Source: CAD feature listing. Evaluate the final solid. Frame: model axes, mm. A direction names the side the tool comes from. Give positions to 0.01 mm unless a question says otherwise; leave off trailing zeros. Loops run counter-clockwise (first coordinate to the right, second up) from the corner with the lowest first, then second, coordinate; pieces in that order, holes last. Notation, with made-up numbers: M -32,29.5 L -9,29.5 A20 ccw -9,40.5 Z; hole C 55.5,1.5 d5. An arc over 180 degrees is marked long. Put each result on its own line as item: value.
Autodesk Inventor part; units mm, degrees
ref_plane "YZ Plane" through (0, 0, 0) normal (1, 0, 0) x (0, 1, 0)
ref_plane "XZ Plane" through (0, 0, 0) normal (0, 1, 0) x (-1, 0, 0)
ref_plane "XY Plane" through (0, 0, 0) normal (0, 0, 1) x (1, 0, 0)
sketch "Sketch1" plane through (0, 0, 0) normal (1, 0, 0) x (0, 1, 0)
  arc A0 (43.0231, 66.0406) -> (13.0231, 66.0406) centre (28.0231, 66.0406) ccw
  arc A1 (13.0231, -33.9594) -> (43.0231, -33.9594) centre (28.0231, -33.9594) ccw
  line L0 (13.0231, 66.0406) -> (13.0231, -33.9594)
  line L1 (43.0231, 66.0406) -> (43.0231, -33.9594)
  circle A2 centre (28.0231, 66.0406) radius 5
  circle A3 centre (28.0231, -33.9594) radius 5
  circle A4 centre (28.0231, 36.0406) radius 2
  circle A5 centre (28.0231, -13.9594) radius 2
  point P0 (0, 0)
  dimension "d6" = 15
  dimension "d18" = 100
  dimension "d40" = 10
  dimension "d50" = 0
  dimension "d51" = 0
  dimension "d52" = 20
  dimension "d53" = 30
  dimension "d54" = 4
  dimension "d66" = 10
extrude "Extrusion6" add sketch "Sketch1" along normal blind 4
hole "Hole4" at (4, 28.0231, 66.0406) direction (-1, 0, 0) diameter 11.6 depth 0.8 tip angle 118
hole "Hole5" at (4, 28.0231, -33.9594) direction (-1, 0, 0) diameter 11.6 depth 0.8
properties part number "BaseJoint"
1. Section query A-A (x = 1.7). Output: boundary loops of the cut face in (y, z).
Found:
outline: M 13.02,-33.96 A15 ccw 43.02,-33.96 L 43.02,66.04 A15 ccw 13.02,66.04 Z; hole C 28.02,-33.96 d10; hole C 28.02,66.04 d10; hole C 28.02,-13.96 d4; hole C 28.02,36.04 d4
2. Contact query for flat-ended pins moving along their axis: P1, Ø2.5, axis at y = 28.02, z = 36.04, coming from the +X side; P2, Ø1.5, axis at x = 1.5, y = 17, coming from the +Z side. Output: stop coordinate, or through.
Found:
P1: through
P2: z = 76.97
3. Section query B-B (y = 15.5). Output: boundary loops of the cut face in (x, z), plus the area to 3 significant figures.
Found:
outline: M 0,-42.22 L 4,-42.22 L 4,74.3 L 0,74.3 Z
area: 466 mm^2
4. Draft query along Z for faces 1 (the cylindrical face through (1.972, 27.693, 81.037)), 2 (the flat face through (4, 28, 17)), 3 (the flat face through (3.2, 23, -36)). Return one class per face: pulls with the +Z half, pulls with the -Z half, needs draft (parallel to the pull), parting line crosses it, or undercut.
Found:
face 1: pulls with the +Z half
face 2: needs draft
face 3: undercut
5. Section query C-C (y = 40.75). Output: boundary loops of the cut face in (x, z), plus the area to 3 significant figures.
Found:
outline: M 0,-41.9 L 4,-41.9 L 4,73.98 L 0,73.98 Z
area: 464 mm^2
6. Material intervals for line 1 (Z direction, x = 1.1, y = 25.25); line 2 (Z direction, x = 0.95, y = 24.75); line 3 (Z direction, x = 2.15, y = 29.5), sorted ascending. Write a range as from..to.
Found:
line 1: -48.7..-38.12, -29.8..61.88, 70.2..80.78
line 2: -48.6..-37.74, -30.18..62.26, 69.82..80.68
line 3: -48.89..-38.74, -29.18..-15.31, -12.61..34.69, 37.39..61.26, 70.82..80.97
7. Access query for faces 4 (the cylindrical face through (3.59, 30.24, -39.32)), 5 (the flat face through (2, 43.023, 17)). Directions: +Z, -Z, +X, -X, +Y, -Y. A direction counts if a zero-diameter tool reaches every point of the face in a straight line with its end or side. Return the directions, or none.
Found:
face 4: +X
face 5: +Z, -Z, +X, -X, +Y
